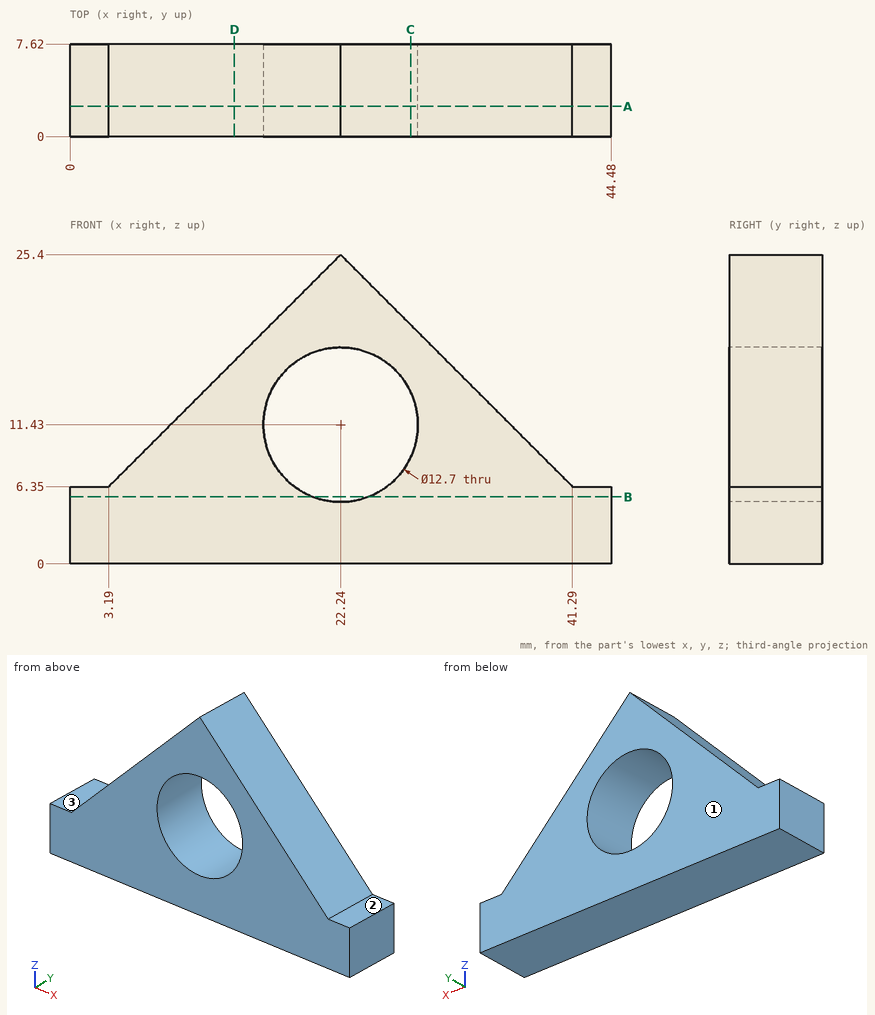
Design review of the part shown in the three views and the two pictorial views. Dimensions are in mm from the part's minimum x, y and z. A direction names the side the tool comes from. Coordinates: 2 decimals unless noted, no trailing zeros. Write each loop counter-clockwise with the first axis right and the second up, starting at its lowest first coordinate (ties: lowest second). Pieces come first, ordered by that corner, then holes.
1) We need section A-A on y = 2.5. State the section outline as (x, z) points, then the cut area to 3 significant figures.
2) We need section D-D on x = 13.5. State the section outline as (y, z) points.
3) We need section C-C on x = 28. State the section outline as (y, z) points, then the cut area to 3 significant figures.
4) Machinability: for the marked faces 1, 2 and 3, which of the approach directions +Z, -Z, +X, -X, +Y, -Y give a long, thin tool a straight path to every point of the face, cutting with its end or side? Answer none if there is none.
5) To check wall thickness, follow probe 1 along Z at (x, y) = (26, 7.25); probe 2 along X at (y, z) = (2.25, 6.25); probe 3 along X at (y, z) = (5.5, 11.43). State the ranges of each line that lie inside material, in increasing order.
6) We need section B-B on z = 5.5. State the section outline as (x, y) points.
7) Clearance check with flat-ended pins moving along their axes: pin 1 Ø2 at (y, z) = (6, 15.5) entering from +X; pin 2 Ø1 at (x, y) = (17, 1.5) entering from +Z; pin 3 Ø3 at (y, z) = (1, 11) entering from +X. State where each tip first meets the part, or that it passes through.
Answer list:
1. outline: (0, 0) - (44.48, 0) - (44.48, 6.35) - (41.29, 6.35) - (22.24, 25.4) - (3.19, 6.35) - (0, 6.35) - close; hole circle Ø12.7 at (22.24, 11.43)
1. area: 519 mm2
2. outline: (0, 0) - (7.62, 0) - (7.62, 16.66) - (0, 16.66) - close
3. outline: (0, 0) - (7.62, 0) - (7.62, 8.76) - (0, 8.76) - close; (0, 14.1) - (7.62, 14.1) - (7.62, 19.64) - (0, 19.64) - close
3. area: 109 mm2
4. face 1: +Z, -Z, +X, -X, +Y
4. face 2: +Z, +X, +Y, -Y
4. face 3: +Z, -X, +Y, -Y
5. probe 1: z = 0 to 6.31, 16.55 to 21.64
5. probe 2: x = 0 to 18.57, 25.91 to 44.48
5. probe 3: x = 8.27 to 15.89, 28.59 to 36.21
6. outline: (0, 0) - (19.97, 0) - (19.97, 7.62) - (0, 7.62) - close; (24.51, 0) - (44.48, 0) - (44.48, 7.62) - (24.51, 7.62) - close
7. pin 1: stops at x = 33.14
7. pin 2: stops at z = 20.66
7. pin 3: stops at x = 38.14
